Could you check a few things on this model? Use its own coordinates, in mm. Coordinates: 2 decimals unless noted, no trailing zeros. Loops run counter-clockwise (first coordinate to the right, second up) from the corner with the lowest first, then second, coordinate; pieces in that order, holes last. Notation, with made-up numbers: M 61,67.25 L 116,67.25 A18 cw 116,98.25 Z; hole C 2.25,-15.5 d4. An arc over 180 degrees is marked long. Return JSON: item names as keys, results as strings. Group by question number.
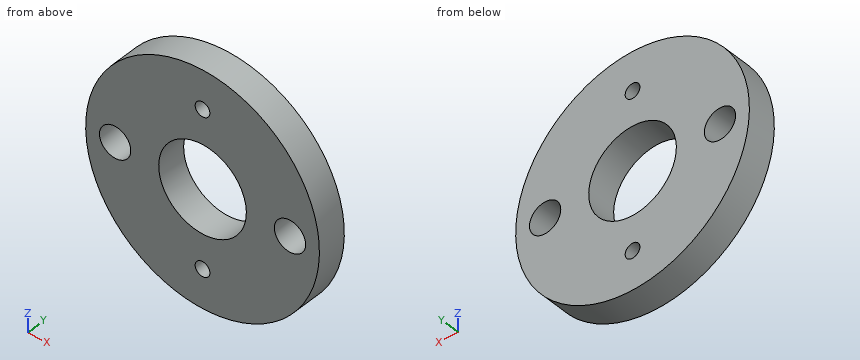
from build123d import *

# Parameters (mm, degrees)
SKETCH1_R                       = 12.7
SKETCH1_R_2                     = 4.7625
BOSS_EXTRUDE1_DEPTH             = 3.175
M3_CLEARANCE_HOLE1_D            = 3.4
M3_CLEARANCE_HOLE1_DEPTH        = 6.35
M3_CLEARANCE_HOLE1_TIP          = 1.021463052
TAP_DRILL_FOR_M2X0_4_TAP1_D     = 1.6
TAP_DRILL_FOR_M2X0_4_TAP1_DEPTH = 6.35
TAP_DRILL_FOR_M2X0_4_TAP1_TIP   = 0.480688495


with BuildPart() as part:
    # Sketch1 → Boss-Extrude1 (new body)
    with BuildSketch(Plane(origin=(0, 0, 0), x_dir=(1, 0, 0), z_dir=(0, 1, 0))):
        with Locations(Location((0, 0, 0), (0, 0, 270))):
            Circle(SKETCH1_R)
        with Locations(Location((0, 0, 0), (0, 0, 270))):
            Circle(SKETCH1_R_2, mode=Mode.SUBTRACT)
    extrude(amount=BOSS_EXTRUDE1_DEPTH)

    # M3 Clearance Hole1
    with Locations(Plane(origin=(0, 3.175, 0), x_dir=(1, 0, 0), z_dir=(0, 1, 0))):
        with Locations((-9.5, 0), (9.5, 0)):
            Hole(M3_CLEARANCE_HOLE1_D / 2, depth=M3_CLEARANCE_HOLE1_DEPTH)
            with Locations((0, 0, -(M3_CLEARANCE_HOLE1_DEPTH + M3_CLEARANCE_HOLE1_TIP / 2))):  # 118° drill point
                Cone(0, M3_CLEARANCE_HOLE1_D / 2, M3_CLEARANCE_HOLE1_TIP, mode=Mode.SUBTRACT)

    # Tap Drill for M2x0.4 Tap1
    with Locations(Plane(origin=(0, 3.175, 0), x_dir=(1, 0, 0), z_dir=(0, 1, 0))):
        with Locations((0, 8.5), (0, -8.5)):
            Hole(TAP_DRILL_FOR_M2X0_4_TAP1_D / 2, depth=TAP_DRILL_FOR_M2X0_4_TAP1_DEPTH)
            with Locations((0, 0, -(TAP_DRILL_FOR_M2X0_4_TAP1_DEPTH + TAP_DRILL_FOR_M2X0_4_TAP1_TIP / 2))):  # 118° drill point
                Cone(0, TAP_DRILL_FOR_M2X0_4_TAP1_D / 2, TAP_DRILL_FOR_M2X0_4_TAP1_TIP, mode=Mode.SUBTRACT)


solid = part.part
(1) Will these pins go through, and if not, where does the flat tip stop? P1, Ø1.5, axis at y = 1.5, z = 10, coming from the -X side; P2, Ø1, axis at y = 3, z = -10, coming from the +X side.
(2) Imagine slicing it at B-B, the plane x = 0. Write out the boundary of the cut face in (y, z) (1 decimal), then the cut area to 3 significant figures.
(3) Imagine slicing it at D-D, the plane x = -9.25. Write out the boundary of the cut face in (y, z) (3 decimals), then the cut area to 3 significant figures.
(4) If I drill on L1, parallel to Z at x = 9.25, y = 0.25; L2, parallel to Z at x = 9, y = 2.6; L3, parallel to X at y = 1.45, z = 3.75, over which ranges is the centre line in solid material (lowest first)? Write a range as [from, to].
(5) Imagine slicing it at A-A, the plane y = 0.4. Write out the boundary of the cut face in (x, z) (1 decimal).
(6) Imagine slicing it at C-C, the plane z = 8.5. Write out the boundary of the cut face in (x, y) (3 decimals), then the cut area to 3 significant figures.
Checks:
{
 "1": {"P1": "x = -8.7", "P2": "x = 8.43"},
 "2": {"outline": "M 0,-12.7 L 3.2,-12.7 L 3.2,-9.3 L 0,-9.3 Z; M 0,-7.7 L 3.2,-7.7 L 3.2,-4.8 L 0,-4.8 Z; M 0,4.8 L 3.2,4.8 L 3.2,7.7 L 0,7.7 Z; M 0,9.3 L 3.2,9.3 L 3.2,12.7 L 0,12.7 Z", "area": "40.2 mm²"},
 "3": {"outline": "M 0,-8.702 L 3.175,-8.702 L 3.175,-1.682 L 0,-1.682 Z; M 0,1.682 L 3.175,1.682 L 3.175,8.702 L 0,8.702 Z", "area": "44.6 mm²"},
 "4": {"L1": "[-8.7, -1.68], [1.68, 8.7]", "L2": "[-8.96, -1.62], [1.62, 8.96]", "L3": "[-12.13, -2.94], [2.94, 12.13]"},
 "5": {"outline": "C 0,0 d25.4; hole C -9.5,0 d3.4; hole C 0,0 d9.5; hole C 0,-8.5 d1.6; hole C 0,8.5 d1.6; hole C 9.5,0 d3.4"},
 "6": {"outline": "M -9.436,0 L -0.8,0 L -0.8,3.175 L -9.436,3.175 Z; M 0.8,0 L 9.436,0 L 9.436,3.175 L 0.8,3.175 Z", "area": "54.8 mm²"}
}
